Verification items for the finished model (mm, model axes). Coordinates: 2 decimals unless noted, no trailing zeros. Write each loop counter-clockwise with the first axis right and the second up, starting at its lowest first coordinate (ties: lowest second). Pieces come first, ordered by that corner, then holes. Notation, with made-up numbers: M 86,6 L 94,6 A26 ccw 94,39 Z; hole C -33.5,12.5 d4. An arc over 180 degrees is marked long. One line per item, written item: value.
Autodesk Inventor part; units mm, degrees
ref_plane "YZ Plane" through (0, 0, 0) normal (1, 0, 0) x (0, 1, 0)
ref_plane "XZ Plane" through (0, 0, 0) normal (0, 1, 0) x (-1, 0, 0)
ref_plane "XY Plane" through (0, 0, 0) normal (0, 0, 1) x (1, 0, 0)
sketch "Sketch1" plane through (0, 0, 0) normal (0, 1, 0) x (-1, 0, 0)
  line L0 (15, 5) -> (-15, 5)
  line L1 (-15, 5) -> (-15, -5)
  line L2 (-15, -5) -> (15, -5)
  line L3 (15, -5) -> (15, 5)
  line L4 (15, 5) -> (-15, -5) construction
  line L5 (-15, 5) -> (15, -5) construction
  circle A0 centre (0, -4) radius 0.5
  line L6 (0, -5) -> (-15, 3)
  line L7 (0, -5) -> (15, 3)
  circle A1 centre (-14, 4) radius 0.5
  circle A2 centre (14, 4) radius 0.5
  point P0 (0, 0)
  dimension "d0" = 30
  dimension "d1" = 10
  dimension "d2" = 1
  dimension "d3" = 1
  dimension "d4" = 2
  dimension "d5" = 2
  dimension "d6" = 1
  dimension "d7" = 1
  dimension "d8" = 1
  dimension "d9" = 1
  dimension "d10" = 1
  dimension "d11" = 1
extrude "Extrusion1" add sketch "Sketch1" along normal blind 1 contours L3 L7 L6 L1 L0
properties part number "bar"
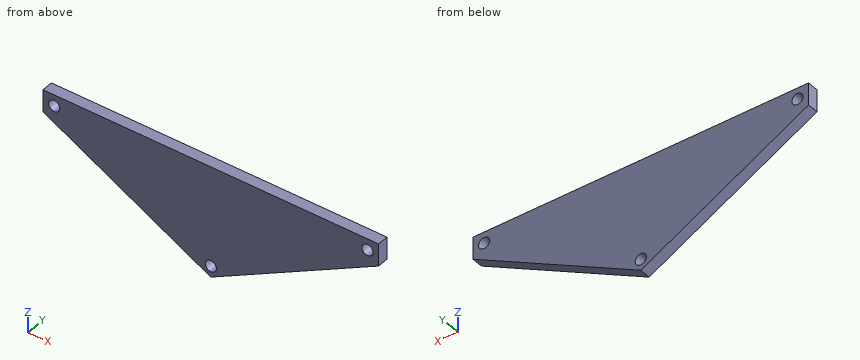
Item 1: Cross-section at C-C, the plane x = -14. Enter the section's corners in (y, z).
The answers:
outline: M 0,2.47 L 1,2.47 L 1,3.5 L 0,3.5 Z; M 0,4.5 L 1,4.5 L 1,5 L 0,5 Z
Item 2: Scan lines: line 1 (Z direction, x = -13, y = 0.2); line 2 (Z direction, x = 7.5, y = 0.4); line 3 (Z direction, x = 14, y = 0.75). Record each from-to range of solid material in increasing order.
The answers:
line 1: z = 1.93 to 5
line 2: z = -1 to 5
line 3: z = 2.47 to 3.5, 4.5 to 5
Item 3: Cross-section at A-A, the plane z = 4. Enter the section's corners in (x, y).
The answers:
outline: M -15,0 L -14.5,0 L -14.5,1 L -15,1 Z; M -13.5,0 L 13.5,0 L 13.5,1 L -13.5,1 Z; M 14.5,0 L 15,0 L 15,1 L 14.5,1 Z
Item 4: Cross-section at B-B, the plane y = 0.3. Enter the section's corners in (x, z).
The answers:
outline: M -15,3 L 0,-5 L 15,3 L 15,5 L -15,5 Z; hole C -14,4 d1; hole C 0,-4 d1; hole C 14,4 d1
Item 5: Cross-section at D-D, the plane z = -4. Enter the section's corners in (x, y) (3 decimals), and give its area (3 significant figures).
The answers:
outline: M -1.875,0 L -0.5,0 L -0.5,1 L -1.875,1 Z; M 0.5,0 L 1.875,0 L 1.875,1 L 0.5,1 Z
area: 2.75 mm²
